Read the model definition and answer for the solid it produces. Units are mm, in the model's axes. Coordinates: 2 decimals unless noted, no trailing zeros. Put each result on its own line as item: value.
from build123d import *

# Parameters (mm, degrees)
CUT_EXTRUDE1_DEPTH = 7.62


with BuildPart() as part:
    # Sketch1 → Revolve1 (revolve)
    with BuildSketch(Plane(origin=(0, 0, 0), x_dir=(0, 0, -1), z_dir=(1, 0, 0))):
        with BuildLine():
            Line((-2.409610907, -44.48919659), (-2.409610907, 6.31080341))
            Line((-2.409610907, 6.31080341), (-1.7653, 6.31080341))
            ThreePointArc((-1.7653, 6.31080341), (0, 4.54550341), (1.7653, 6.31080341))
            Line((1.7653, 6.31080341), (2.409610907, 6.31080341))
            Line((2.409610907, 6.31080341), (2.409610907, -44.48919659))
            Line((2.409610907, -44.48919659), (-2.409610907, -44.48919659))
        make_face()
    revolve(axis=Axis((0, -47.02919659, 19.251181834), (0, 0, -1)))

    # Sketch2 → Cut-Extrude1 (cut)
    with BuildSketch(Plane(origin=(0, 0, -2.409610907), x_dir=(-1, 0, 0), z_dir=(0, 0, -1))):
        with BuildLine():
            Line((-9.161557863, -0.373493478), (9.161557863, -0.373493478))
            ThreePointArc((9.161557863, -0.373493478), (11.176404431, -1.366886448), (11.615239648, -3.570034182))
            Line((11.615239648, -3.570034182), (3.310434261, -34.607484824))
            ThreePointArc((3.310434261, -34.607484824), (2.403359506, -35.965790688), (0.856752476, -36.490944119))
            Line((0.856752476, -36.490944119), (-0.856752476, -36.490944119))
            ThreePointArc((-0.856752476, -36.490944119), (-2.403359506, -35.965790688), (-3.310434261, -34.607484824))
            Line((-3.310434261, -34.607484824), (-11.615239648, -3.570034182))
            ThreePointArc((-11.615239648, -3.570034182), (-11.176404431, -1.366886448), (-9.161557863, -0.373493478))
        make_face()
        with BuildLine():
            Line((38.943483164, -24.512142867), (11.124307138, -40.586550481))
            ThreePointArc((11.124307138, -40.586550481), (9.52244114, -40.905619058), (8.057485269, -40.183342291))
            Line((8.057485269, -40.183342291), (6.845854298, -38.971711321))
            ThreePointArc((6.845854298, -38.971711321), (6.123577532, -37.506755449), (6.442646109, -35.904889451))
            Line((6.442646109, -35.904889451), (22.517053723, -8.085713426))
            ThreePointArc((22.517053723, -8.085713426), (24.385217783, -6.838156081), (26.512364361, -7.560432847))
            Line((26.512364361, -7.560432847), (39.468763743, -20.516832229))
            ThreePointArc((39.468763743, -20.516832229), (40.191040509, -22.643978806), (38.943483164, -24.512142867))
        make_face()
        with BuildLine():
            Line((43.459162408, -58.644436238), (12.421711766, -50.339630851))
            ThreePointArc((12.421711766, -50.339630851), (11.063405902, -49.432556096), (10.53825247, -47.885949066))
            Line((10.53825247, -47.885949066), (10.53825247, -46.172444114))
            ThreePointArc((10.53825247, -46.172444114), (11.063405902, -44.625837084), (12.421711766, -43.718762329))
            Line((12.421711766, -43.718762329), (43.459162408, -35.413956942))
            ThreePointArc((43.459162408, -35.413956942), (45.662310142, -35.852792158), (46.655703112, -37.867638727))
            Line((46.655703112, -37.867638727), (46.655703112, -56.190754453))
            ThreePointArc((46.655703112, -56.190754453), (45.662310142, -58.205601021), (43.459162408, -58.644436238))
        make_face()
        with BuildLine():
            Line((22.517053723, -85.972679753), (6.442646109, -58.153503728))
            ThreePointArc((6.442646109, -58.153503728), (6.123577532, -56.55163773), (6.845854298, -55.086681859))
            Line((6.845854298, -55.086681859), (8.057485269, -53.875050888))
            ThreePointArc((8.057485269, -53.875050888), (9.52244114, -53.152774122), (11.124307138, -53.471842699))
            Line((11.124307138, -53.471842699), (38.943483164, -69.546250313))
            ThreePointArc((38.943483164, -69.546250313), (40.191040509, -71.414414373), (39.468763743, -73.54156095))
            Line((39.468763743, -73.54156095), (26.512364361, -86.497960333))
            ThreePointArc((26.512364361, -86.497960333), (24.385217783, -87.220237099), (22.517053723, -85.972679753))
        make_face()
        with BuildLine():
            Line((-11.615239648, -90.488358998), (-3.310434261, -59.450908356))
            ThreePointArc((-3.310434261, -59.450908356), (-2.403359506, -58.092602492), (-0.856752476, -57.56744906))
            Line((-0.856752476, -57.56744906), (0.856752476, -57.56744906))
            ThreePointArc((0.856752476, -57.56744906), (2.403359506, -58.092602492), (3.310434261, -59.450908356))
            Line((3.310434261, -59.450908356), (11.615239648, -90.488358998))
            ThreePointArc((11.615239648, -90.488358998), (11.176404431, -92.691506732), (9.161557863, -93.684899702))
            Line((9.161557863, -93.684899702), (-9.161557863, -93.684899702))
            ThreePointArc((-9.161557863, -93.684899702), (-11.176404431, -92.691506732), (-11.615239648, -90.488358998))
        make_face()
        with BuildLine():
            Line((-38.943483164, -69.546250313), (-11.124307138, -53.471842699))
            ThreePointArc((-11.124307138, -53.471842699), (-9.52244114, -53.152774122), (-8.057485269, -53.875050888))
            Line((-8.057485269, -53.875050888), (-6.845854298, -55.086681859))
            ThreePointArc((-6.845854298, -55.086681859), (-6.123577532, -56.55163773), (-6.442646109, -58.153503728))
            Line((-6.442646109, -58.153503728), (-22.517053723, -85.972679753))
            ThreePointArc((-22.517053723, -85.972679753), (-24.385217783, -87.220237099), (-26.512364361, -86.497960333))
            Line((-26.512364361, -86.497960333), (-39.468763743, -73.54156095))
            ThreePointArc((-39.468763743, -73.54156095), (-40.191040509, -71.414414373), (-38.943483164, -69.546250313))
        make_face()
        with BuildLine():
            Line((-43.459162408, -35.413956942), (-12.421711766, -43.718762329))
            ThreePointArc((-12.421711766, -43.718762329), (-11.063405902, -44.625837084), (-10.53825247, -46.172444114))
            Line((-10.53825247, -46.172444114), (-10.53825247, -47.885949066))
            ThreePointArc((-10.53825247, -47.885949066), (-11.063405902, -49.432556096), (-12.421711766, -50.339630851))
            Line((-12.421711766, -50.339630851), (-43.459162408, -58.644436238))
            ThreePointArc((-43.459162408, -58.644436238), (-45.662310142, -58.205601021), (-46.655703112, -56.190754453))
            Line((-46.655703112, -56.190754453), (-46.655703112, -37.867638727))
            ThreePointArc((-46.655703112, -37.867638727), (-45.662310142, -35.852792158), (-43.459162408, -35.413956942))
        make_face()
        with BuildLine():
            Line((-22.517053723, -8.085713426), (-6.442646109, -35.904889451))
            ThreePointArc((-6.442646109, -35.904889451), (-6.123577532, -37.506755449), (-6.845854298, -38.971711321))
            Line((-6.845854298, -38.971711321), (-8.057485269, -40.183342291))
            ThreePointArc((-8.057485269, -40.183342291), (-9.52244114, -40.905619058), (-11.124307138, -40.586550481))
            Line((-11.124307138, -40.586550481), (-38.943483164, -24.512142867))
            ThreePointArc((-38.943483164, -24.512142867), (-40.191040509, -22.643978806), (-39.468763743, -20.516832229))
            Line((-39.468763743, -20.516832229), (-26.512364361, -7.560432847))
            ThreePointArc((-26.512364361, -7.560432847), (-24.385217783, -6.838156081), (-22.517053723, -8.085713426))
        make_face()
    extrude(amount=-CUT_EXTRUDE1_DEPTH, mode=Mode.SUBTRACT)


solid = part.part
Q1. Given pin 1 (2.5 mm diameter, centred on y = -43.5, z = 1, fed in from -X); pin 2 (0.5 mm diameter, centred on x = 0.5, z = 0.5, fed in from +Y); pin 3 (0.9 mm diameter, centred on y = -47.5, z = -0.5, fed in from +X), each flat-ended and moving along its own axis, determine where each tip first touches the part or whether it passes through.
Answers below:
pin 1: stops at x = -53.28
pin 2: stops at y = 4.71
pin 3: stops at x = 51.85
Q2. Consider line 1 along X through (y, z) = (-72, 0.05); line 2 along X through (y, z) = (-61, -1.15); line 3 along Y through (x, z) = (2, -0.45). Determine where each line is inside the solid, lowest interval first.
Answers below:
line 1: x = -45.13 to -40.2, -14.44 to -6.67, 6.67 to 14.44, 40.2 to 45.13
line 2: x = -50.09 to -24.15, -8.09 to -3.72, 3.72 to 8.09, 24.15 to 50.09
line 3: y = -98.62 to -93.68, -57.84 to -48.59, -45.46 to -36.22, -0.37 to 4.57
Q3. For a pull along Y with two mould halves and no side action, classify faces 1 (the face through (46.656, -47, 0)), 2 (the face through (16.02, 3.85, -2.09)), 3 (the face through (-11, -24, -2.41)) as +Y half, -Y half, draft (parallel to the pull), parting line (faces both ways), or undercut.
Answers below:
face 1: undercut
face 2: parting line
face 3: draft
Q4. Find section A-A on x = 17. Give the number of separate pieces and of enclosed holes in the cut face, plus the area to 3 significant figures.
Answers below:
separate pieces: 4
enclosed holes: 0
area: 245 mm^2
